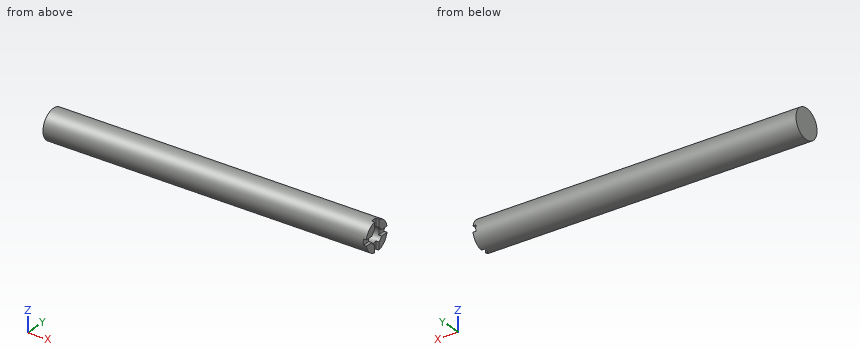
from build123d import *

# Parameters (mm, degrees)
F0_R     = 12.7
F1_DEPTH = 279.4
F2_R     = 6.35
F3_DEPTH = 25.4
F5_DEPTH = 2.54


with BuildPart() as f1:
    # F0 (on Right) → F1 (new body)
    with BuildSketch(Plane.YZ):
        Circle(F0_R)
    extrude(amount=F1_DEPTH)

    # F2 (on face) → F3 (cut)
    with BuildSketch(Plane.YZ.offset(279.4)):
        Circle(F2_R)
    extrude(amount=-F3_DEPTH, mode=Mode.SUBTRACT)

    # F4 (on face) → F5 (cut)
    with BuildSketch(Plane.YZ.offset(279.4)):
        with BuildLine():
            Line((-5.8198711326, 2.54), (-12.4434078933, 2.54))
            ThreePointArc((-12.4434078933, 2.54), (-12.6356891432, 1.2764638175), (-12.7, 0))
            ThreePointArc((-12.7, 0), (-12.6356891432, -1.2764638175), (-12.4434078933, -2.54))
            Line((-12.4434078933, -2.54), (-5.8198711326, -2.54))
            ThreePointArc((-5.8198711326, -2.54), (-6.35, 0), (-5.8198711326, 2.54))
        make_face()
        with BuildLine():
            Line((12.4434078933, 2.54), (5.8198711326, 2.54))
            ThreePointArc((5.8198711326, 2.54), (6.2160550871, 1.2973662374), (6.35, 0))
            ThreePointArc((6.35, 0), (6.2160550871, -1.2973662374), (5.8198711326, -2.54))
            Line((5.8198711326, -2.54), (12.4434078933, -2.54))
            ThreePointArc((12.4434078933, -2.54), (12.6356891432, -1.2764638175), (12.7, 0))
            ThreePointArc((12.7, 0), (12.6356891432, 1.2764638175), (12.4434078933, 2.54))
        make_face()
        with BuildLine():
            ThreePointArc((0, 12.7), (-1.2764638175, 12.6356891432), (-2.54, 12.4434078933))
            Line((-2.54, 12.4434078933), (-2.54, 5.8198711326))
            ThreePointArc((-2.54, 5.8198711326), (0, 6.35), (2.54, 5.8198711326))
            Line((2.54, 5.8198711326), (2.54, 12.4434078933))
            ThreePointArc((2.54, 12.4434078933), (1.2764638175, 12.6356891432), (0, 12.7))
        make_face()
        with BuildLine():
            Line((-2.54, -5.8198711326), (-2.54, -12.4434078933))
            ThreePointArc((-2.54, -12.4434078933), (-1.2764638175, -12.6356891432), (0, -12.7))
            ThreePointArc((0, -12.7), (1.2764638175, -12.6356891432), (2.54, -12.4434078933))
            Line((2.54, -12.4434078933), (2.54, -5.8198711326))
            ThreePointArc((2.54, -5.8198711326), (0, -6.35), (-2.54, -5.8198711326))
        make_face()
    extrude(amount=-F5_DEPTH, mode=Mode.SUBTRACT)


solid = f1.part
For this review, take the finished solid that the model builds, in its own axes (mm). Coordinates: 2 decimals unless noted, no trailing zeros. Loops run counter-clockwise (first coordinate to the right, second up) from the corner with the lowest first, then second, coordinate; pieces in that order, holes last. Notation, with made-up numbers: (31.25, -14.75) - (78.25, -14.75) arc R23 ccw to (78.25, 2.25) - close; hole circle Ø2 at (39.5, -35.5). An arc over 180 degrees is marked (long way). Use a Markdown table: item, result. Add a question column.
Item 1: For line 1 (Z direction, x = 269.5, y = 0); line 2 (Y direction, x = 141, z = 2.25), list the stretches that pass through material, from the lowest coordinate up.
Item 2: We need section C-C (x = 44). Give the boundary of the cut face in (y, z), and give its area (3 significant figures).
Item 3: We need section A-A (y = 0). Give the boundary of the cut face in (x, z).
Item 4: Insertion check: pin 1 Ø1.5 at (y, z) = (0, 11) entering from +X; pin 2 Ø5.5 at (y, z) = (-9, -0.5) entering from +X; pin 3 Ø3 at (x, z) = (277.5, -10.5) entering from +Y; pin 4 Ø4 at (y, z) = (-1, 1.5) entering from +X. Each pin has a flat end and moves straight along its axis. Give the tip position at first contact, or say it passes through.
Results list:
| question | item | result |
|---|---|---|
| 1 | line 1 | z = -12.7 to -6.35, 6.35 to 12.7 |
| 1 | line 2 | y = -12.5 to 12.5 |
| 2 | outline | circle Ø25.4 at (0, 0) |
| 2 | area | 507 mm^2 |
| 3 | outline | (0, -12.7) - (276.86, -12.7) - (276.86, -6.35) - (254, -6.35) - (254, 6.35) - (276.86, 6.35) - (276.86, 12.7) - (0, 12.7) - close |
| 4 | pin 1 | stops at x = 276.86 |
| 4 | pin 2 | stops at x = 279.4 |
| 4 | pin 3 | stops at y = 8.96 |
| 4 | pin 4 | stops at x = 254 |
